For this review, use the dimensioned drawing (mm, ordinates from the lowest corner) and the shaded views. A direction names the side the tool comes from. Give positions to 0.01 mm unless a question says otherwise; leave off trailing zeros. Order: outer loops, then holes, each group sorted by start corner. A loop starts at its lowest first (then second) coordinate and runs counter-clockwise, first axis right, second up. Notation, with made-up numbers: (-32.5, 12) -> (19.5, 12) arc R28 cw to (19.5, 51) -> close; hole circle Ø2 at (68, -30). An arc over 180 degrees is marked (long way). One line per item, written item: value. Start each with the question number.
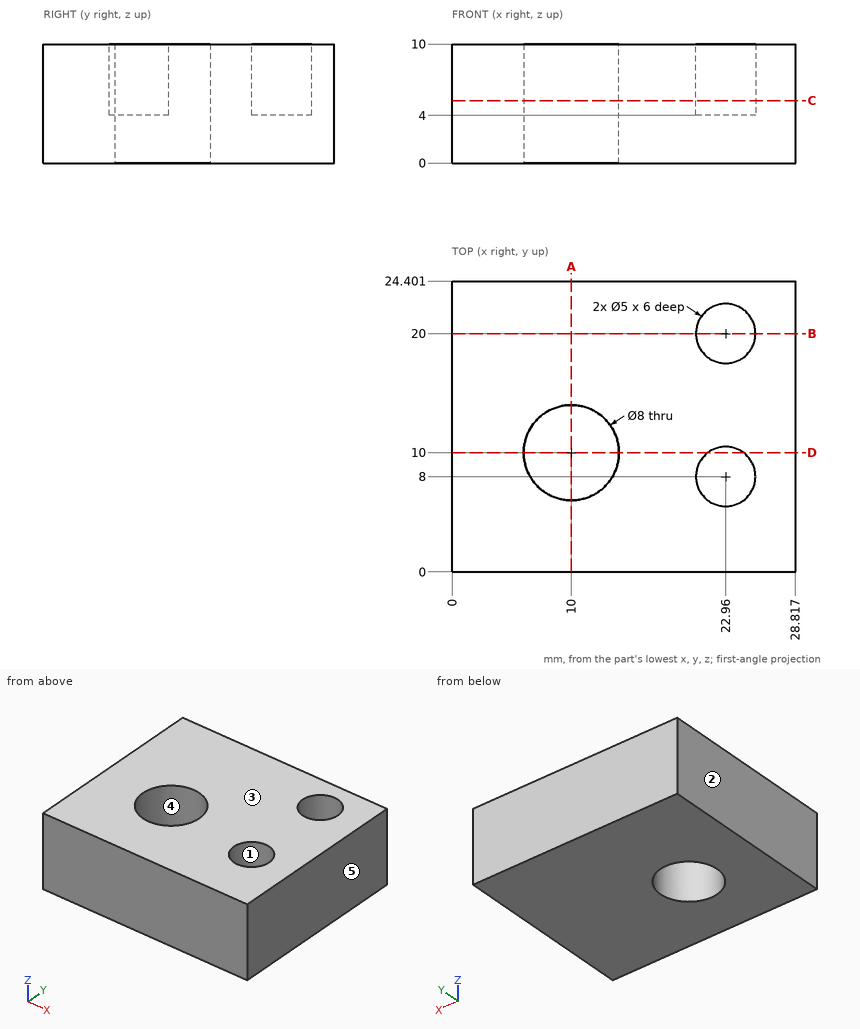
Q1. For pin 1 Ø1.5 at (x, y) = (24, 7) entering from +Z; pin 2 Ø4.5 at (x, y) = (22.96, 8) entering from -Z, all flat-tipped, find the tip position at first contact; note any pin that passes through.
Q2. Take a section at C-C (z = 5.25). State the section outline as (x, y) points.
Q3. Take a section at B-B (y = 20). State the section outline as (x, z) points.
Q4. Mouldability with a two-part tool opening along X and no side actions: class the marked faces 3, 4 and 5 as pulls with the +X half, pulls with the -X half, needs draft (parallel to the pull), parting line crosses it, or undercut.
Q5. For line 1 along Y through (x, z) = (21.25, 8) (1 decimal); line 2 along Y through (x, z) = (10, 3.5); line 3 along Z through (x, y) = (22.5, 7.25), list the stretches that pass through material, from the lowest coordinate up.
Q6. Take a section at A-A (x = 10). State the section outline as (y, z) points, and give its area (3 significant figures).
Q7. Take a section at D-D (y = 10). State the section outline as (x, z) points, and give its area (3 significant figures).
Q8. For the marked faces 1 and 2, list the 3-axis set-ups (+Z, -Z, +X, -X, +Y, -Y) from which the entire face can be reached by the end or side of a thin tool; tool diameter is ignored.
Answers below:
1. pin 1: stops at z = 4
1. pin 2: stops at z = 0
2. outline: (0, 0) -> (28.82, 0) -> (28.82, 24.4) -> (0, 24.4) -> close; hole circle Ø8 at (10, 10); hole circle Ø5 at (22.96, 8); hole circle Ø5 at (22.96, 20)
3. outline: (0, 0) -> (28.82, 0) -> (28.82, 10) -> (25.46, 10) -> (25.46, 4) -> (20.46, 4) -> (20.46, 10) -> (0, 10) -> close
4. face 3: needs draft
4. face 4: undercut
4. face 5: pulls with the +X half
5. line 1: y = 0 to 6.2, 9.8 to 18.2, 21.8 to 24.4
5. line 2: y = 0 to 6, 14 to 24.4
5. line 3: z = 0 to 4
6. outline: (0, 0) -> (6, 0) -> (6, 10) -> (0, 10) -> close; (14, 0) -> (24.4, 0) -> (24.4, 10) -> (14, 10) -> close
6. area: 164 mm²
7. outline: (0, 0) -> (6, 0) -> (6, 10) -> (0, 10) -> close; (14, 0) -> (28.82, 0) -> (28.82, 10) -> (24.46, 10) -> (24.46, 4) -> (21.46, 4) -> (21.46, 10) -> (14, 10) -> close
7. area: 190 mm²
8. face 1: +Z
8. face 2: +Z, -Z, -X, +Y, -Y
